from build123d import *

# Parameters (mm, degrees)
SKETCH1_W           = 76.2
SKETCH1_H           = 51.562
BOSS_EXTRUDE1_DEPTH = 6.35
SKETCH2_W           = 27.94
SKETCH2_H           = 12.7
CUT_EXTRUDE1_DEPTH  = 9.906
FILLET1_R           = 5.08
SKETCH7_R           = 2.75
CUT_EXTRUDE2_DEPTH  = 127
CUT_EXTRUDE4_DEPTH  = 32.416
SKETCH9_W           = 27.94
SKETCH9_H           = 20
CUT_EXTRUDE5_DEPTH  = 18.7
FILLET2_R           = 5.1
SKETCH10_R          = 1.5
CUT_EXTRUDE6_DEPTH  = 10


with BuildPart() as part:
    # Sketch1 → Boss-Extrude1 (new body)
    with BuildSketch(Plane.XY):
        with Locations((38.1, 25.781)):
            Rectangle(SKETCH1_W, SKETCH1_H)
    extrude(amount=BOSS_EXTRUDE1_DEPTH)

    # Sketch2 → Cut-Extrude1 (cut)
    with BuildSketch(Plane.XY.offset(6.35)):
        with Locations((38.1, 45.212)):
            Rectangle(SKETCH2_W, SKETCH2_H)
    extrude(amount=-CUT_EXTRUDE1_DEPTH, mode=Mode.SUBTRACT)

    # Fillet1
    fillet1_edges = [part.edges().sort_by_distance(p)[0] for p in [
        (0, 51.562, 3.175),
        (76.2, 51.562, 3.175),
    ]]
    fillet(fillet1_edges, radius=FILLET1_R)

    # Sketch7 → Cut-Extrude2 (cut)
    with BuildSketch(Plane(origin=(0, 0, 0), x_dir=(-1, 0, 0), z_dir=(0, 0, -1))):
        with Locations((-11.588, 16.8)):
            Circle(SKETCH7_R)
        with Locations((-64.612, 16.8)):
            Circle(SKETCH7_R)
    extrude(amount=-CUT_EXTRUDE2_DEPTH, mode=Mode.SUBTRACT)

    # Sketch8 → Cut-Extrude4 (cut)
    with BuildSketch(Plane.XY.offset(6.35)):
        with BuildLine():
            ThreePointArc((64.612, 43.312), (61.862, 40.562), (64.612, 37.812))
            Line((64.612, 37.812), (64.612, 40.562))
            Line((64.612, 40.562), (64.612, 43.312))
        make_face()
        with BuildLine():
            Line((64.612, 40.562), (64.612, 37.812))
            ThreePointArc((64.612, 37.812), (66.556543648, 38.617456352), (67.362, 40.562))
            ThreePointArc((67.362, 40.562), (66.556543648, 42.506543648), (64.612, 43.312))
            Line((64.612, 43.312), (64.612, 40.562))
        make_face()
    cut_extrude4 = extrude(amount=-CUT_EXTRUDE4_DEPTH, mode=Mode.SUBTRACT)

    # Mirror2: Cut-Extrude4 across plane
    add(cut_extrude4.mirror(Plane.ZY.offset(-38.1)), mode=Mode.SUBTRACT)

    # Sketch9 → Cut-Extrude5 (cut)
    with BuildSketch(Plane.XY.offset(6.35)):
        with Locations((38.1, 28.862)):
            Rectangle(SKETCH9_W, SKETCH9_H)
    extrude(amount=-CUT_EXTRUDE5_DEPTH, mode=Mode.SUBTRACT)

    # Fillet2
    fillet2_edges = [part.edges().sort_by_distance(p)[0] for p in [
        (52.07, 51.562, 3.175),
        (24.13, 51.562, 3.175),
        (52.07, 18.862, 3.175),
        (24.13, 18.862, 3.175),
    ]]
    fillet(fillet2_edges, radius=FILLET2_R)

    # Sketch10 → Cut-Extrude6 (cut)
    with BuildSketch(Plane.XY.offset(6.35)):
        with Locations((47.98, 13.83)):
            Circle(SKETCH10_R)
        with Locations((28.1, 13.83)):
            Circle(SKETCH10_R)
    extrude(amount=-CUT_EXTRUDE6_DEPTH, mode=Mode.SUBTRACT)


solid = part.part
Model file for the job. Use its own axes, mm. A direction names the side the tool comes from. Give positions to 0.01 mm unless a question says otherwise; leave off trailing zeros. Order: outer loops, then holes, each group sorted by start corner. A loop starts at its lowest first (then second) coordinate and runs counter-clockwise, first axis right, second up. Notation, with made-up numbers: M 47,53.5 L 55,53.5 A5 ccw 55,61.5 Z; hole C -31.75,13.25 d6. An arc over 180 degrees is marked long. Put each result on its own line as item: value. Start each with the question number.
(1) Band-saw the part on B-B on y = 16.8. Give the cut face in (x, z).
(2) Pin check, flat tip, straight feed: pin 1 Ø1.9 at (x, z) = (41.5, 3.5) entering from +Y. Stop position of the tip, or through.
(3) Band-saw the part on A-A on y = 37. Give the cut face in (x, z).
(4) Tool access for faces 1 (the face through (25.58, 20.4, 3.13)), 2 (the face through (12, 51.562, 3)): list every direction of +Z, -Z, +X, -X, +Y, -Y with a clear straight run to the whole face (end or side of a thin tool).
(5) Pull direction Y, two halves, no side cores. Call faces 3 (the face through (26.99, 14.84, 3.22)), 4 (the face through (52.07, 35, 3)), 5 (the face through (38, 18.862, 3)): released by +Y, released by -Y, zero draft, split by the parting line, or undercut.
(6) Drill centre lines: L1, parallel to X at y = 45, z = 1.25; L2, parallel to X at y = 15, z = 4; L3, parallel to X at y = 12.5, z = 4.5. Where is each one in solid material? Low to high. Write a range as [from, to].
(7) Band-saw the part on D-D on x = 54. Give the cut face in (y, z), then the cut area to 3 significant figures.
(8) Band-saw the part on C-C on x = 28.1. Give the cut face in (y, z), then the cut area to 3 significant figures.
Results below:
1. outline: M 0,0 L 8.84,0 L 8.84,6.35 L 0,6.35 Z; M 14.34,0 L 61.86,0 L 61.86,6.35 L 14.34,6.35 Z; M 67.36,0 L 76.2,0 L 76.2,6.35 L 67.36,6.35 Z
2. pin 1: stops at y = 18.86
3. outline: M 0,0 L 24.13,0 L 24.13,6.35 L 0,6.35 Z; M 52.07,0 L 76.2,0 L 76.2,6.35 L 52.07,6.35 Z
4. face 1: +Z, -Z, +Y
4. face 2: +Z, -Z, +X, -X, +Y
5. face 3: undercut
5. face 4: zero draft
5. face 5: released by +Y
6. L1: x = [0, 24.13], [52.07, 76.2]
6. L2: x = [0, 9.51], [13.67, 27.16], [29.04, 47.04], [48.92, 62.53], [66.69, 76.2]
6. L3: x = [0, 27.41], [28.79, 47.29], [48.67, 76.2]
7. outline: M 0,0 L 50.46,0 L 50.46,6.35 L 0,6.35 Z
7. area: 320 mm2
8. outline: M 0,0 L 12.33,0 L 12.33,6.35 L 0,6.35 Z; M 15.33,0 L 18.99,0 L 18.99,6.35 L 15.33,6.35 Z
8. area: 102 mm2
